Study the drawing (mm; zero at the part's minimum x, y, z) and answer. A direction names the side the tool comes from. Coordinates: 2 decimals unless noted, no trailing zeros. Loops run counter-clockwise (first coordinate to the right, second up) from the corner with the lowest first, then second, coordinate; pieces in that order, holes last. Notation, with made-up numbers: (5, 71) - (57, 71) arc R19 ccw to (57, 86) - close; hole circle Ø6 at (-24.75, -40). An arc over 180 degrees is marked (long way). Write each question's results on one line, items separated by ' | '. Start each with the question number.
(1) Find section A-A on z = 7. Determine the outline of the cut face in (x, y).
(2) For the marked faces 1 and 2, determine the directions among +Z, -Z, +X, -X, +Y, -Y from which every point of the face is accessible in a straight line to the end or side of a thin tool.
(3) Given pin 1 Ø5 at (y, z) = (15, 7.5) entering from +X; pin 2 Ø5 at (x, z) = (32.5, 3) entering from -Y, each flat-ended and moving along its own axis, determine where each tip first touches the part or whether it passes through.
(4) Consider line 1 (X direction, y = 21.5, z = 1.75); line 2 (Y direction, x = 29.5, z = 5.75). Determine where each line is inside the solid, lowest interval first. Write a range as from..to.
(5) Find section C-C on y = 11.5. Determine the outline of the cut face in (x, z), then the cut area to 3 significant figures.
(6) Find section B-B on x = 41.5. Determine the outline of the cut face in (y, z).
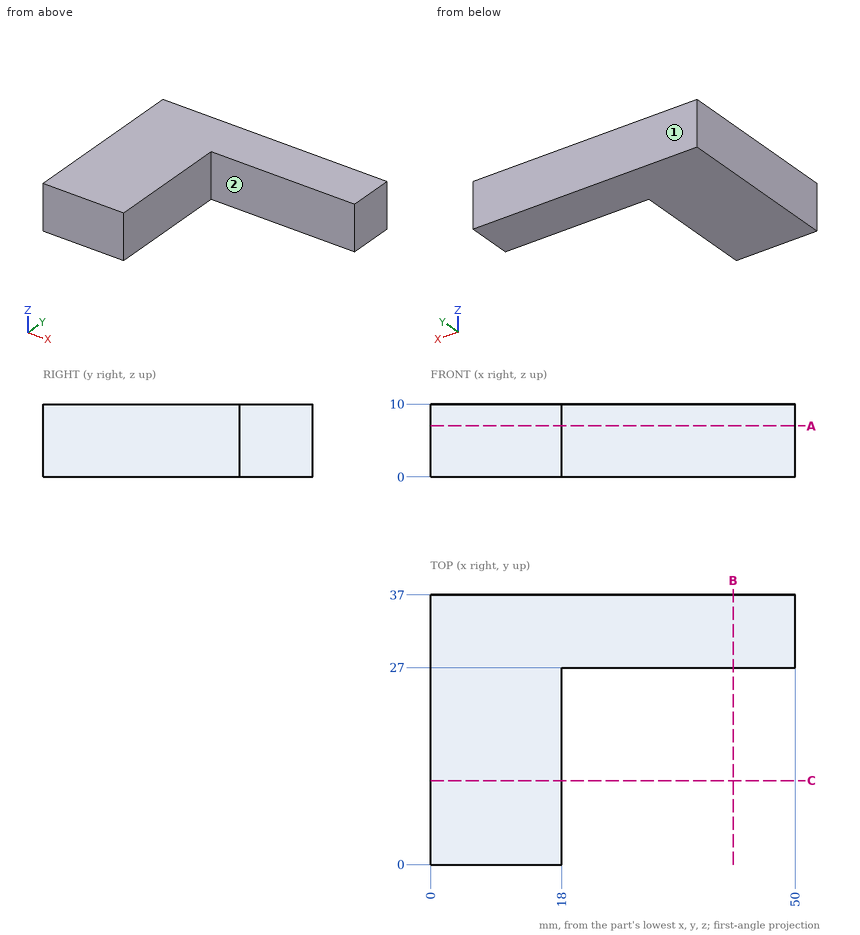
Values:
1) outline: (0, 0) - (18, 0) - (18, 27) - (50, 27) - (50, 37) - (0, 37) - close
2) face 1: +Z, -Z, +X, -X, +Y | face 2: +Z, -Z, +X, -Y
3) pin 1: stops at x = 18 | pin 2: stops at y = 27
4) line 1: x = 0..18 | line 2: y = 27..37
5) outline: (0, 0) - (18, 0) - (18, 10) - (0, 10) - close | area: 180 mm²
6) outline: (27, 0) - (37, 0) - (37, 10) - (27, 10) - close
